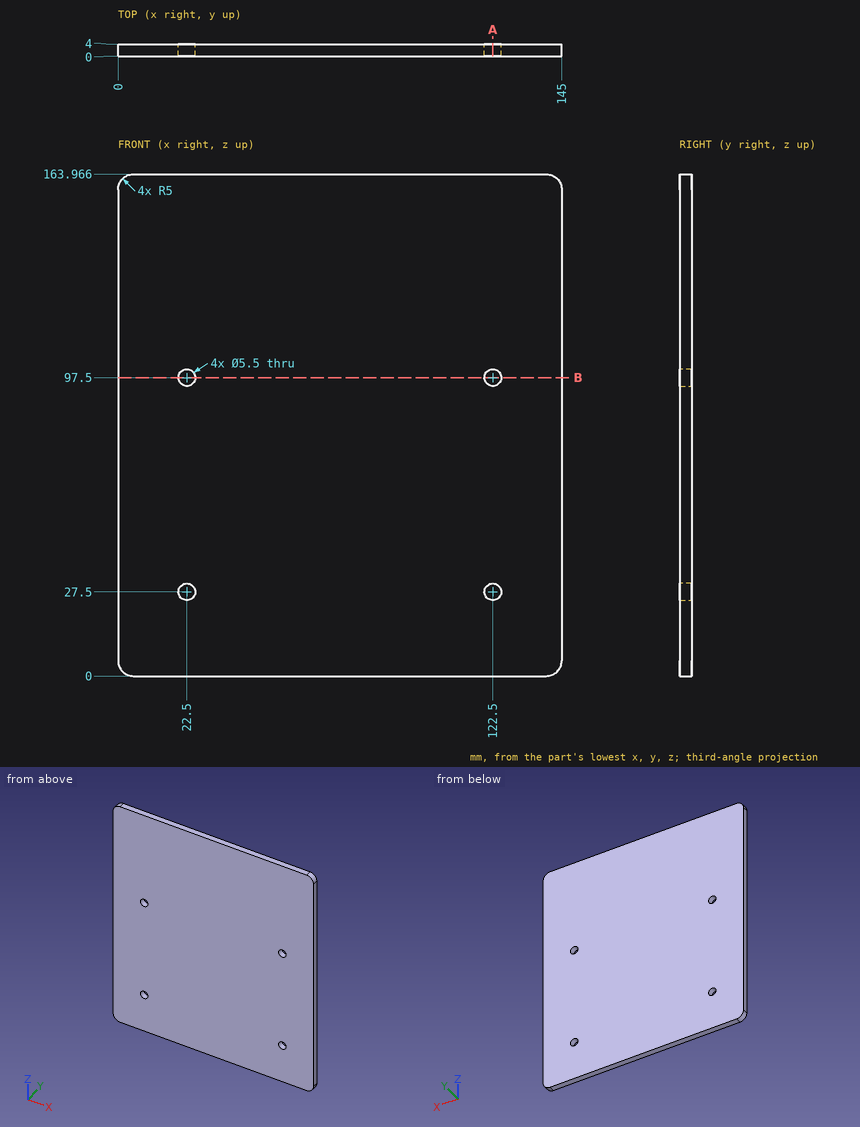
Can you work these out from the drawing? Everything is in mm from the part's minimum corner. Coordinates: 2 decimals unless noted, no trailing zeros. Loops run counter-clockwise (first coordinate to the right, second up) from the corner with the lowest first, then second, coordinate; pieces in that order, holes last. Notation, with made-up numbers: M -27,35.25 L 14,35.25 A25 ccw 14,71.25 Z; hole C -18,60.25 d5. An arc over 180 degrees is marked long. Put each result on its own line as item: value. Start each with the question number.
(1) Suppose I cut it at A-A on x = 122.5. Please give me the cut outline in (y, z).
(2) Will this pin go through, and if not, where does the flat tip stop? P1, Ø5, axis at x = 122.5, z = 27.5, coming from the -Y side.
(3) Suppose I cut it at B-B on z = 97.5. Please give me the cut outline in (x, y).
(4) I need wall thicknesses on line 1 (X direction, y = 0.9, z = 97.5); line 2 (X direction, y = 1.2, z = 96.5). Which ranges of each line are inside material? Lowest first, please. Write a range as from..to.
Solutions:
1. outline: M 0,0 L 4,0 L 4,24.75 L 0,24.75 Z; M 0,30.25 L 4,30.25 L 4,94.75 L 0,94.75 Z; M 0,100.25 L 4,100.25 L 4,163.97 L 0,163.97 Z
2. P1: passes through
3. outline: M 0,0 L 19.75,0 L 19.75,4 L 0,4 Z; M 25.25,0 L 119.75,0 L 119.75,4 L 25.25,4 Z; M 125.25,0 L 145,0 L 145,4 L 125.25,4 Z
4. line 1: x = 0..19.75, 25.25..119.75, 125.25..145
4. line 2: x = 0..19.94, 25.06..119.94, 125.06..145
